Input: part model. Units: mm. Frame: model coordinates. A direction names the side the tool comes from. Give positions to 0.01 mm unless a question says otherwise; leave off trailing zeros. Loops run counter-clockwise (first coordinate to the right, second up) from the corner with the lowest first, then second, coordinate; pieces in that order, holes last. Notation, with made-up numbers: (87, 54) - (114, 54) arc R24 ccw to (114, 84) - close; hole circle Ø4 at (60.5, 0.25). An arc over 180 degrees is marked (long way). One line per question, with ' | ' between items. Start each with the question number.
from build123d import *

# Parameters (mm, degrees)
SKETCH_1_W               = 80
SKETCH_1_H               = 25
EXTRUDE_1_DEPTH          = 1
SM_START                 = -12.5
SM_EDGE_FLANGE_1_DEPTH   = 25
SM_EDGE_FLANGE_1_2_DEPTH = 25
SM_EDGE_FLANGE_2_DEPTH   = 25
SM_EDGE_FLANGE_2_2_DEPTH = 25
SKETCH_18_R              = 1.5
CUT_EXTRUDE_1_DEPTH      = 1
SKETCH_19_R              = 1.5
CUT_EXTRUDE_2_DEPTH      = 1


# Read off the part's stored shape, not the designer's step: Ребро-кромка1, Ребро-кромка2
with BuildPart() as part:
    # Sketch 1 → Бобышка-Вытянуть1 (new body)
    with BuildSketch(Plane(origin=(0, 0, 0), x_dir=(1, 0, 0), z_dir=(0, 1, 0))):
        Rectangle(SKETCH_1_W, SKETCH_1_H)
    extrude(amount=EXTRUDE_1_DEPTH)

    # Ребро-кромка1 outline → Ребро-кромка1 (cut)
    with BuildSketch(Plane.XY.offset(SM_START)):
        with BuildLine():
            Line((-40, 0), (-39.977477944, 0))
            ThreePointArc((-39.977477944, 0), (-39.429289785, 0.724744872), (-38.563264381, 1))
            Line((-38.563264381, 1), (-40, 1))
            Line((-40, 1), (-40, 0))
        make_face()
        with BuildLine():
            Line((40, 1), (38.563264381, 1))
            ThreePointArc((38.563264381, 1), (39.429289785, 0.724744872), (39.977477944, 0))
            Line((39.977477944, 0), (40, 0))
            Line((40, 0), (40, 1))
        make_face()
    extrude(amount=SM_EDGE_FLANGE_1_DEPTH, mode=Mode.SUBTRACT)

    # Sm Edge Flange 1 2 outline → Sm Edge Flange 1 2 (add)
    with BuildSketch(Plane.XY.offset(SM_START)):
        with BuildLine():
            ThreePointArc((-39.977477944, 0), (-40.015252138, -0.123527486), (-40.042258437, -0.24984688))
            Line((-40.042258437, -0.24984688), (-54.339743625, -84.781655225))
            Line((-54.339743625, -84.781655225), (-53.353747587, -84.948423972))
            Line((-53.353747587, -84.948423972), (-39.0562624, -0.416615627))
            ThreePointArc((-39.0562624, -0.416615627), (-38.885993225, -0.118101986), (-38.563264381, 0))
            Line((-38.563264381, 0), (-39.977477944, 0))
        make_face()
        with BuildLine():
            Line((39.977477944, 0), (38.563264381, 0))
            ThreePointArc((38.563264381, 0), (38.885993225, -0.118101986), (39.0562624, -0.416615627))
            Line((39.0562624, -0.416615627), (53.353747587, -84.948423972))
            Line((53.353747587, -84.948423972), (54.339743625, -84.781655225))
            Line((54.339743625, -84.781655225), (40.042258437, -0.24984688))
            ThreePointArc((40.042258437, -0.24984688), (40.015252138, -0.123527486), (39.977477944, 0))
        make_face()
    extrude(amount=SM_EDGE_FLANGE_1_2_DEPTH)

    # Ребро-кромка2 outline → Ребро-кромка2 (cut)
    with BuildSketch(Plane.XY.offset(SM_START)):
        with BuildLine():
            Line((54.339743625, -84.781655225), (54.33598765, -84.759448567))
            ThreePointArc((54.33598765, -84.759448567), (53.529971426, -84.339802009), (53.114144989, -83.531808345))
            Line((53.114144989, -83.531808345), (53.353747587, -84.948423972))
            Line((53.353747587, -84.948423972), (54.339743625, -84.781655225))
        make_face()
        with BuildLine():
            ThreePointArc((-53.114144989, -83.531808345), (-53.529971426, -84.339802009), (-54.33598765, -84.759448567))
            Line((-54.33598765, -84.759448567), (-54.339743625, -84.781655225))
            Line((-54.339743625, -84.781655225), (-53.353747587, -84.948423972))
            Line((-53.353747587, -84.948423972), (-53.114144989, -83.531808345))
        make_face()
    extrude(amount=SM_EDGE_FLANGE_2_DEPTH, mode=Mode.SUBTRACT)

    # Sm Edge Flange 2 2 outline → Sm Edge Flange 2 2 (add)
    with BuildSketch(Plane.XY.offset(SM_START)):
        with BuildLine():
            ThreePointArc((54.33598765, -84.759448567), (54.464084816, -84.776093249), (54.593139045, -84.781655225))
            Line((54.593139045, -84.781655225), (63.325540765, -84.781655225))
            Line((63.325540765, -84.781655225), (63.325540765, -83.781655225))
            Line((63.325540765, -83.781655225), (54.593139045, -83.781655225))
            ThreePointArc((54.593139045, -83.781655225), (54.270410201, -83.663553239), (54.100141026, -83.365039598))
            Line((54.100141026, -83.365039598), (54.33598765, -84.759448567))
        make_face()
        with BuildLine():
            Line((-63.325540765, -83.781655225), (-63.325540765, -84.781655225))
            Line((-63.325540765, -84.781655225), (-54.593139045, -84.781655225))
            ThreePointArc((-54.593139045, -84.781655225), (-54.464084816, -84.776093249), (-54.33598765, -84.759448567))
            Line((-54.33598765, -84.759448567), (-54.100141026, -83.365039598))
            ThreePointArc((-54.100141026, -83.365039598), (-54.270410201, -83.663553239), (-54.593139045, -83.781655225))
            Line((-54.593139045, -83.781655225), (-63.325540765, -83.781655225))
        make_face()
    extrude(amount=SM_EDGE_FLANGE_2_2_DEPTH)

    # Эскиз18 → Вырез-Вытянуть1 (cut)
    with BuildSketch(Plane(origin=(0, 1, 0), x_dir=(1, 0, 0), z_dir=(0, 1, 0))):
        with Locations(Location((-7.563264381, 7.5, 0), (0, 0, 270))):
            Circle(SKETCH_18_R)
        with Locations(Location((-7.563264381, -7.5, 0), (0, 0, 90))):
            Circle(SKETCH_18_R)
    extrude(amount=-CUT_EXTRUDE_1_DEPTH, mode=Mode.SUBTRACT)

    # Эскиз19 → Вырез-Вытянуть2 (cut)
    with BuildSketch(Plane(origin=(0, -83.781655225, 0), x_dir=(1, 0, 0), z_dir=(0, 1, 0))):
        with Locations(Location((58.325540765, 7.5, 0), (0, 0, 270))):
            Circle(SKETCH_19_R)
        with Locations(Location((58.325540765, -7.5, 0), (0, 0, 90))):
            Circle(SKETCH_19_R)
        with Locations(Location((-58.325540765, -7.5, 0), (0, 0, 270))):
            Circle(SKETCH_19_R)
        with Locations(Location((-58.325540765, 7.5, 0), (0, 0, 90))):
            Circle(SKETCH_19_R)
    extrude(amount=-CUT_EXTRUDE_2_DEPTH, mode=Mode.SUBTRACT)


solid = part.part
Q1. Draft query along Z for faces 1 (the face through (-56.84, -84.27, 7.3)), 2 (the face through (-59.813, -84.275, -7.305)), 3 (the face through (-1, 1, 0)). Return one class per face: +Z half, -Z half, draft (parallel to the pull), parting line (faces both ways), or undercut.
Q2. Section C-C, the plane x = 28. Output: boundary loops of the cut face in (y, z).
Q3. Section D-D, the plane x = 46. Output: boundary loops of the cut face in (y, z), plus the area to 3 significant figures.
Q4. Section B-B, the plane z = -7.5. Count the separate pieces of the cut face and the enclosed holes in it, plus the area to 3 significant figures.
Q5. Access query for faces 4 (the face through (59, -83.782, 0)), 5 (the face through (59.813, -84.275, -7.695)), 6 (the face through (-59, -83.782, 0)), 7 (the face through (-1, 0, 0)). Directions: +Z, -Z, +X, -X, +Y, -Y. A direction counts if a zero-diameter tool reaches every point of the face in a straight line with its end or side. Return the directions, or none.
Q6. Section A-A, the plane y = -10.5. Output: boundary loops of the cut face in (x, z), plus the area to 3 significant figures.
Q7. First-contact query: pin 1 (2.5 mm diameter, centred on x = 60, z = 0, fed in from +Y); pin 2 (2.5 mm diameter, centred on x = 58.33, z = 7.5, fed in from -Y); pin 3 (2 mm diameter, centred on y = -48.5, z = 10, fed in from +X); pin 4 (4 mm diameter, centred on y = -46, z = 5.5, fed in from -X). Flat tips, straight axial feed; report the tip coordinate or a pass-through.
Q8. Line query: L1, parallel to Y at x = 29, z = 6.5; L2, parallel to X at y = -84.1, z = 7.5; L3, parallel to X at y = 0.2, z = 7.5. Output: solid intervals per line, ascending. Write a range as from..to.
Solved:
1) face 1: undercut | face 2: undercut | face 3: draft
2) outline: (0, -12.5) - (1, -12.5) - (1, 12.5) - (0, 12.5) - close
3) outline: (-41.47, -12.5) - (-35.47, -12.5) - (-35.47, 12.5) - (-41.47, 12.5) - close | area: 150 mm²
4) separate pieces: 4 | enclosed holes: 0 | area: 260 mm²
5) face 4: +Z, -Z, +X, +Y | face 5: +Y, -Y | face 6: +Z, -Z, -X, +Y | face 7: +Z, -Z, -Y
6) outline: (-41.78, -12.5) - (-40.76, -12.5) - (-40.76, 12.5) - (-41.78, 12.5) - close; (40.76, -12.5) - (41.78, -12.5) - (41.78, 12.5) - (40.76, 12.5) - close | area: 50.7 mm²
7) pin 1: stops at y = -83.78 | pin 2: passes through | pin 3: stops at x = 48.37 | pin 4: stops at x = -48.12
8) L1: y = 0..1 | L2: x = -63.33..-59.83, -56.83..-53.34, 53.34..56.83, 59.83..63.33 | L3: x = -39.89..-9.06, -6.06..39.89
